Check sheet for the modelled part. Datum: model origin and axes. Units: mm. A direction names the side the tool comes from. Round coordinates to 2 decimals unless told otherwise and drop trailing zeros. Write each loop counter-clockwise with the first axis right and the second up, starting at its lowest first coordinate (ties: lowest second). Pieces come first, ordered by that corner, then holes. Notation, with made-up numbers: (1, 53) -> (26, 53) arc R19 ccw to (26, 80) -> close; hole circle Ø2 at (-8.75, 14.25). An arc over 180 degrees is marked (long way). One line per item, written item: value.
Autodesk Inventor part; units mm, degrees
ref_plane "YZ Plane" through (0, 0, 0) normal (1, 0, 0) x (0, 1, 0)
ref_plane "XZ Plane" through (0, 0, 0) normal (0, 1, 0) x (-1, 0, 0)
ref_plane "XY Plane" through (0, 0, 0) normal (0, 0, 1) x (1, 0, 0)
sketch "Esboço1" plane through (0, 0, 0) normal (0, 0, 1) x (1, 0, 0)
  circle A0 centre (0, 51.901) radius 2.4
  circle A1 centre (0, 19.901) radius 2.4
  circle A2 centre (-32, 19.901) radius 2.4
  line L0 (-36, 3.901) -> (-36, 51.901)
  circle A3 centre (0, 19.901) radius 4
  circle A4 centre (0, 51.901) radius 4
  circle A5 centre (-32, 19.901) radius 4
  line L1 (-36, 15.901) -> (0, 15.901)
  line L2 (4, 19.901) -> (4, 51.901)
  line L3 (0, 55.901) -> (-36, 55.901)
  line L4 (-36, 55.901) -> (-36, 15.901)
  circle A6 centre (-32, 51.901) radius 4
  circle A7 centre (-32, 51.901) radius 2.4
  point P0 (0, 0)
  point P1 (-36, 19.901)
  point P2 (-32, 15.901)
  point P3 (-32, 55.901)
  dimension "d0" = 8
  dimension "d1" = 8
  dimension "d2" = 8
  dimension "d12" = 8
extrude "Extrusão1" add sketch "Esboço1" along normal blind 3.25 contours L0 A6 L3 A4 L2 A3 L1 A5 | A5 | A6 | A3 | A4
sketch "Esboço2" plane through (0, 0, 3.25) normal (0, 0, 1) x (1, 0, 0)
  arc A0 (-22.6, 24.751) -> (-22.45, 24.601) centre (-22.45, 24.751) ccw
  line L0 (-0.3, 39.0723) -> (-0.3, 24.751)
  line L1 (-4.4, 47.201) -> (-0.45, 47.201)
  line L2 (-0.3, 24.601) -> (-0.3, 47.201)
  line L3 (-22.6, 47.201) -> (-22.6, 24.601)
  line L4 (1.7, 49.201) -> (1.7, 22.601)
  line L5 (-24.6, 22.601) -> (-24.6, 47.201)
  line L6 (-22.6, 47.201) -> (-24.6, 47.201)
  line L7 (-7, 49.201) -> (-7, 47.201)
  line L8 (-4.4, 49.201) -> (-4.4, 47.201)
  line L9 (-4.4, 24.601) -> (-4.4, 22.601)
  line L10 (-7, 24.601) -> (-7, 22.601)
  line L11 (-22.6, 24.601) -> (-7, 24.601)
  line L12 (-4.4, 24.601) -> (-0.3, 24.601)
  line L13 (1.7, 22.601) -> (-4.4, 22.601)
  line L14 (-7, 22.601) -> (-24.6, 22.601)
  line L15 (-16, 49.201) -> (-7, 49.201)
  line L16 (-4.4, 49.201) -> (1.7, 49.201)
  line L17 (-0.3, 47.201) -> (-4.4, 47.201)
  line L18 (-7, 47.201) -> (-16, 47.201)
  line L19 (-16, 47.201) -> (-16, 49.201)
  point P0 (0, 0)
extrude "Extrusão2" add sketch "Esboço2" along normal blind 12.25 contours L3 L11 L10 L14 L5 L6 | L2 L17 L1 L8 L16 L4 L13 L9 L12 L0 | L7 L18 L19 L15
sketch "Esboço3" plane through (1.7, 22.601, 3.25) normal (1, 0, 0) x (0, 0, -1)
  arc A0 (-6.15, 9.8) -> (-3.3, 12.65) centre (-6.15, 12.65) ccw
  line L0 (-3.3, 12.8939) -> (-3.3, 12.65)
  line L1 (-6.15, 9.8) -> (-12.25, 9.8)
  line L2 (-12.25, 24.6) -> (-12.25, 0)
  line L3 (0, 24.6) -> (-12.25, 24.6)
  line L4 (-6.15, 24.6) -> (-12.25, 24.6)
  arc A1 (-3.3, 12.8939) -> (-6.15, 24.6) centre (-6.15, 18.4) ccw
  point P0 (3.25, -22.601)
extrude "Extrusão3" cut sketch "Esboço3" against normal blind 12.25
sketch "Esboço4" plane through (0, 0, 0) normal (0, 0, -1) x (-1, 0, 0)
  circle A0 centre (0, 19.901) radius 2.4
  circle A1 centre (32, 19.901) radius 2.4
  circle A2 centre (0, 51.901) radius 2.4
  circle A3 centre (32, 51.901) radius 2.4
  circle A4 centre (32, 51.901) radius 3.1
  circle A5 centre (0, 51.901) radius 3.1
  circle A6 centre (0, 19.901) radius 3.1
  circle A7 centre (32, 19.901) radius 3.1
  point P0 (0, 0)
extrude "Extrusão4" cut sketch "Esboço4" against normal blind 1
properties part number "apoio servo"
Item 1: Tool access check on faces 4 (the cylindrical face through (-29.54, 50.015, 0.493)), 5 (the flat face through (-1, 49.201, 9)), 6 (the flat face through (-4.4, 48, 9)), 7 (the flat face through (-16, 22.601, 9)). Record the directions out of +Z, -Z, +X, -X, +Y, -Y that give a thin tool (end or side, any length) a straight path to the whole face; none if there is none.
Answer:
face 4: -Z
face 5: +Z, +X, -X, +Y
face 6: +Z, +Y, -Y
face 7: +Z, +X, -X, -Y
Item 2: Depth check by flat-ended pin: P1, Ø8, axis at x = -8.5, y = 33.5, coming from the -Z side; P2, Ø6, axis at y = 28.5, z = 6.5, coming from the +X side; P3, Ø3, axis at x = 0, z = 9.5, coming from the -Y side; P4, Ø3, axis at x = -32, y = 51.901, coming from the -Z side. Enter the tip coordinate at first touch or a pass-through.
Answer:
P1: stops at z = 0
P2: stops at x = 1.7
P3: stops at y = 22.6
P4: passes through
Item 3: Sectioned sample at A-A on y = 51. Enter the section's corners in (x, z), and give its area (3 significant figures).
Answer:
outline: (-36, 0) -> (-34.97, 0) -> (-34.97, 1) -> (-34.22, 1) -> (-34.22, 3.25) -> (-36, 3.25) -> close; (-29.78, 1) -> (-29.03, 1) -> (-29.03, 0) -> (-2.97, 0) -> (-2.97, 1) -> (-2.22, 1) -> (-2.22, 3.25) -> (-29.78, 3.25) -> close; (2.22, 1) -> (2.97, 1) -> (2.97, 0) -> (4, 0) -> (4, 3.25) -> (2.22, 3.25) -> close
area: 98.1 mm^2
Item 4: Sectioned sample at B-B on z = 4. Enter the section's corners in (x, y).
Answer:
outline: (-24.6, 22.6) -> (-7, 22.6) -> (-7, 24.6) -> (-22.6, 24.6) -> (-22.6, 47.2) -> (-24.6, 47.2) -> close; (-16, 47.2) -> (-7, 47.2) -> (-7, 49.2) -> (-16, 49.2) -> close; (-4.4, 22.6) -> (1.7, 22.6) -> (1.7, 37.95) -> (-0.3, 37.95) -> (-0.3, 24.6) -> (-4.4, 24.6) -> close; (-4.4, 47.2) -> (-0.3, 47.2) -> (-0.3, 44.05) -> (1.7, 44.05) -> (1.7, 49.2) -> (-4.4, 49.2) -> close
Item 5: Mould release check, pull along X, two halves, no side actions. Record for faces 1 (the cylindrical face through (-1.22, 41.22, 3.204)), 2 (the cylindrical face through (0.71, 33.21, 7.41)), 3 (the flat face through (-24.6, 35, 9)): pulls with the +X half, pulls with the -X half, needs draft (parallel to the pull), parting line crosses it, or undercut.
Answer:
face 1: undercut
face 2: needs draft
face 3: pulls with the -X half
Item 6: Sectioned sample at D-D on y = 41. Enter the section's corners in (x, z), and give its area (3 significant figures).
Answer:
outline: (-36, 0) -> (4, 0) -> (4, 3.25) -> (1.7, 3.25) -> (1.7, 3.2) -> (-10.55, 3.2) -> (-10.55, 3.25) -> (-22.6, 3.25) -> (-22.6, 15.5) -> (-24.6, 15.5) -> (-24.6, 3.25) -> (-36, 3.25) -> close
area: 154 mm^2
Item 7: Sectioned sample at C-C on x = -12. Enter the section's corners in (y, z).
Answer:
outline: (15.9, 0) -> (55.9, 0) -> (55.9, 3.25) -> (49.2, 3.25) -> (49.2, 15.5) -> (47.2, 15.5) -> (47.2, 3.25) -> (24.6, 3.25) -> (24.6, 15.5) -> (22.6, 15.5) -> (22.6, 3.25) -> (15.9, 3.25) -> close
Item 8: Thickness scan on line 1 (Y direction, x = 0, z = 0.6); line 2 (Y direction, x = -32, z = 2.4); line 3 (X direction, y = 32, z = 10). Record the ranges inside material, lowest first.
Answer:
line 1: y = 15.9 to 16.8, 23 to 48.8, 55 to 55.9
line 2: y = 15.9 to 17.5, 22.3 to 49.5, 54.3 to 55.9
line 3: x = -24.6 to -22.6, -0.3 to 1.7
